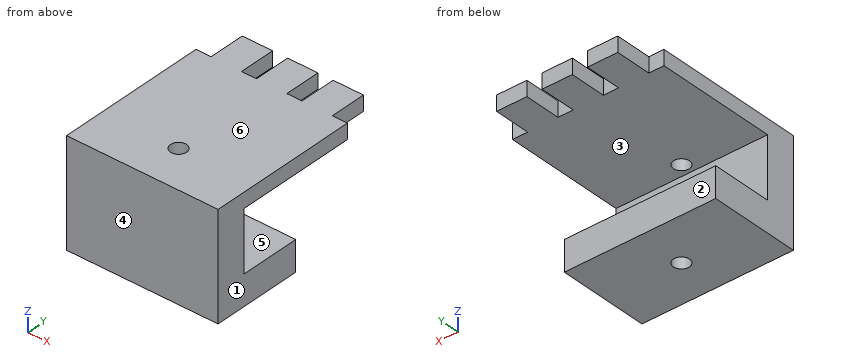
Autodesk Inventor part; units mm, degrees
ref_plane "YZ Plane" through (0, 0, 0) normal (1, 0, 0) x (0, 1, 0)
ref_plane "XZ Plane" through (0, 0, 0) normal (0, 1, 0) x (-1, 0, 0)
ref_plane "XY Plane" through (0, 0, 0) normal (0, 0, 1) x (1, 0, 0)
sketch "Sketch1" plane through (0, 0, 0) normal (0, 0, 1) x (1, 0, 0)
  line L0 (69.608, 72.6391) -> (69.608, 22.6391)
  line L1 (69.608, 22.6391) -> (19.608, 22.6391)
  line L2 (19.608, 22.6391) -> (19.608, 72.6391)
  line L3 (19.608, 72.6391) -> (24.608, 72.6391)
  line L4 (24.608, 72.6391) -> (24.608, 84.6391)
  line L5 (24.608, 84.6391) -> (34.608, 84.6391)
  line L6 (34.608, 84.6391) -> (34.608, 72.6391)
  line L7 (34.608, 72.6391) -> (39.608, 72.6391)
  line L8 (39.608, 72.6391) -> (39.608, 84.6391)
  line L9 (39.608, 84.6391) -> (49.608, 84.6391)
  line L10 (49.608, 84.6391) -> (49.608, 72.6391)
  line L11 (49.608, 72.6391) -> (54.608, 72.6391)
  line L12 (54.608, 72.6391) -> (54.608, 84.6391)
  line L13 (54.608, 84.6391) -> (64.608, 84.6391)
  line L14 (64.608, 84.6391) -> (64.608, 72.6391)
  line L15 (64.608, 72.6391) -> (69.608, 72.6391)
  point P0 (0, 0)
  dimension "d0" = 50
  dimension "d1" = 50
  dimension "d2" = 5
  dimension "d3" = 12
  dimension "d4" = 10
  dimension "d5" = 12
  dimension "d6" = 5
  dimension "d7" = 12
  dimension "d8" = 10
  dimension "d9" = 12
  dimension "d10" = 5
  dimension "d11" = 12
  dimension "d12" = 10
  dimension "d13" = 12
  dimension "d14" = 5
extrude "Extrusion1" add sketch "Sketch1" along normal blind 5
sketch "Sketch2" plane through (69.608, 22.6391, 0) normal (1, 0, 0) x (0, 0, -1)
  line L0 (0, 50) -> (0, 0)
  line L1 (0, 0) -> (30, 0)
  line L2 (30, 0) -> (30, 25)
  line L3 (30, 25) -> (20, 25)
  line L4 (20, 25) -> (20, 10)
  line L5 (20, 10) -> (0, 10)
  point P0 (0, -22.6391)
  dimension "d17" = 30
  dimension "d18" = 25
  dimension "d19" = 10
  dimension "d20" = 15
  dimension "d21" = 20
sketch "Sketch3" plane through (0, 0, 5) normal (0, 0, 1) x (1, 0, 0)
  point P0 (0, 0)
extrude "Extrusion2" add sketch "Sketch2" against normal blind 50
sketch "Sketch4" plane through (69.608, 22.6391, 5) normal (1, 0, 0) x (0, 0, -1)
  line L0 (35, 25) -> (25, 25)
  line L1 (35, 25) -> (35, 30)
  line L2 (35, 25) -> (35, 0)
  line L3 (35, 30) -> (25, 30)
  line L4 (25, 30) -> (25, 25)
  line L5 (25, 25) -> (35, 25)
  point P0 (5, -22.6391)
  dimension "d24" = 5
  dimension "d25" = 10
  dimension "d26" = 5
  dimension "d27" = 10
extrude "Extrusion3" add sketch "Sketch4" against normal blind 50
sketch "Sketch5" plane through (69.608, 22.6391, 5) normal (1, 0, 0) x (0, 0, -1)
  point P0 (5, -22.6391)
sketch "Sketch6" plane through (0, 0, 5) normal (0, 0, 1) x (1, 0, 0)
  line L0 (69.608, 22.6391) -> (19.608, 22.6391)
  circle A0 centre (44.608, 36.6391) radius 2.65
  point P0 (0, 0)
  dimension "d31" = 5.3
extrude "Extrusion4" cut sketch "Sketch6" against normal blind 50
sketch "Sketch7" plane through (69.608, 22.6391, 5) normal (1, 0, 0) x (0, 0, -1)
  point P0 (5, -22.6391)
sketch "Sketch8" plane through (0, 0, 5) normal (0, 0, 1) x (1, 0, 0)
  point P0 (0, 0)
sketch "Sketch9" plane through (69.608, 22.6391, 5) normal (1, 0, 0) x (0, 0, -1)
  point P0 (5, -22.6391)
sketch "Sketch10" plane through (69.608, 22.6391, 5) normal (1, 0, 0) x (0, 0, -1)
  point P0 (5, -22.6391)
properties part number "Casis Kiri Roda"
Geometry: final body of the model. Coordinates: model frame, mm. Face numbers are marked on the shaded views. A direction names the side the tool comes from. Give positions to 0.01 mm unless a question says otherwise; leave off trailing zeros. Loops run counter-clockwise (first coordinate to the right, second up) from the corner with the lowest first, then second, coordinate; pieces in that order, holes last. Notation, with made-up numbers: M 6,18.5 L 41,18.5 A31 ccw 41,46.5 Z; hole C 8,13 d4. An arc over 180 degrees is marked long. Put each result on its own line as item: value. Start each with the question number.
1) Cut plane A-A (y = 77). Output: boundary loops of the cut face in (x, z).
2) Cut plane D-D (z = -3). Output: boundary loops of the cut face in (x, y), then the cut area to 3 significant figures.
3) Access query for the marked faces 1, 2 and 3. Directions: +Z, -Z, +X, -X, +Y, -Y. A direction counts if a zero-diameter tool reaches every point of the face in a straight line with its end or side. Return the directions, or none.
4) Cut plane B-B (x = 66). Output: boundary loops of the cut face in (y, z).
5) Contact query for flat-ended pins moving along their axis: pin 1 (2.5 mm diameter, centred on y = 78, z = 1.5, fed in from -X); pin 2 (1 mm diameter, centred on x = 46, z = -1, fed in from +Y); pin 3 (11 mm diameter, centred on x = 51, z = -27, fed in from +Y); pin 4 (5 mm diameter, centred on x = 44.61, y = 36.64, fed in from -Z). Output: stop coordinate, or through.
6) Pull-direction query (Z, two-part tool) for the marked faces 4, 5 and 6; classes: pulls with the +Z half, pulls with the -Z half, needs draft (parallel to the pull), parting line crosses it, or undercut.
7) Ray query, line 1 along Z through (x, y) = (43, 42); line 2 along Y through (x, z) = (36.5, -17); line 3 along Z through (x, y) = (47, 80). Return the intervals inside material, ascending.
8) Cut plane C-C (z = -23.5). Output: boundary loops of the cut face in (x, y), then the cut area to 3 significant figures.
Verdict:
1. outline: M 24.61,0 L 34.61,0 L 34.61,5 L 24.61,5 Z; M 39.61,0 L 49.61,0 L 49.61,5 L 39.61,5 Z; M 54.61,0 L 64.61,0 L 64.61,5 L 54.61,5 Z
2. outline: M 19.61,22.64 L 69.61,22.64 L 69.61,32.64 L 19.61,32.64 Z
2. area: 500 mm2
3. face 1: +Z, -Z, +X, +Y, -Y
3. face 2: -Z, +X, -X, +Y
3. face 3: +X, -X, +Y
4. outline: M 22.64,-30 L 52.64,-30 L 52.64,-20 L 32.64,-20 L 32.64,0 L 72.64,0 L 72.64,5 L 22.64,5 Z
5. pin 1: x = 24.61
5. pin 2: y = 32.64
5. pin 3: y = 52.64
5. pin 4: through
6. face 4: needs draft
6. face 5: undercut
6. face 6: pulls with the +Z half
7. line 1: -30 to -20, 0 to 5
7. line 2: 22.64 to 32.64
7. line 3: 0 to 5
8. outline: M 19.61,22.64 L 69.61,22.64 L 69.61,52.64 L 19.61,52.64 Z; hole C 44.61,36.64 d5.3
8. area: 1,480 mm2
